Input: part model. Units: mm. Frame: model coordinates. Coordinates: 2 decimals unless noted, no trailing zeros. Loops run counter-clockwise (first coordinate to the right, second up) from the corner with the lowest first, then second, coordinate; pieces in that order, holes last. Notation, with made-up numbers: (34, 17.5) - (61, 17.5) arc R14 ccw to (61, 22.5) - close; hole circle Ø4 at (31.25, 3.25). An arc over 180 degrees is marked (long way). Use a Markdown table: item, result. Add a question column.
1. Ray query, L1, parallel to Y at x = 8.5, z = 2.05; L2, parallel to Y at x = -21.5, z = 2.85; L3, parallel to Y at x = 86, z = 1.1. Return the intervals inside material, ascending. Write a range as [from, to].
2. Section query B-B on x = 14. Return the cut outline in (y, z), then the cut area to 3 significant figures.
3. Section query D-D on x = -55.5. Return the cut outline in (y, z).
4. Contact query for flat-ended pins moving along their axis: P1, Ø1.5, axis at y = 71.5, z = 1, coming from the -X side; P2, Ø0.8, axis at x = 1, z = 1.5, coming from the +Y side. Output: stop coordinate, or through.
5. Section query C-C on x = -29. Return the cut outline in (y, z).
6. Draft query along Y for faces 1 (the face through (127.673, -116.235, 1.454)), 2 (the face through (76.285, 57.453, 1.454)), 3 (the face through (12, -34, 2.95)). Return one class per face: released by +Y, released by -Y, zero draft, split by the parting line, or undercut.
7. Section query A-A on z = 1.7. Return the cut outline in (x, y), then the cut area to 3 significant figures.
```python
from build123d import *

# Parameters (mm, degrees)
SKETCH1_W           = 15.45
SKETCH1_H           = 6.08
BOSS_EXTRUDE1_DEPTH = 2.95


with BuildPart() as part:
    # Sketch1 → Boss-Extrude1 (new body)
    with BuildSketch(Plane.XY):
        with BuildLine():
            Line((0.171167624, 69.469671818), (2.671167624, 69.469671818))
            Line((2.671167624, 69.469671818), (2.671167624, 75.099671818))
            Line((2.671167624, 75.099671818), (17.671167624, 75.099671818))
            Line((17.671167624, 75.099671818), (17.671167624, 69.469671818))
            Line((17.671167624, 69.469671818), (20.171167624, 69.469671818))
            ThreePointArc((20.171167624, 69.469671818), (77.092371221, 57.340494982), (135.171167624, 53.599671818))
            Line((135.171167624, 53.599671818), (135.171167624, -108.900328182))
            ThreePointArc((135.171167624, -108.900328182), (127.671167624, -116.400328182), (135.171167624, -123.900328182))
            Line((135.171167624, -123.900328182), (135.171167624, -146.400328182))
            Line((135.171167624, -146.400328182), (-114.828832376, -146.400328182))
            Line((-114.828832376, -146.400328182), (-114.828832376, 53.599671818))
            ThreePointArc((-114.828832376, 53.599671818), (-56.750035973, 57.340494982), (0.171167624, 69.469671818))
        make_face()
        with Locations((10.171167624, 50.559671818)):
            Rectangle(SKETCH1_W, SKETCH1_H, mode=Mode.SUBTRACT)
    extrude(amount=BOSS_EXTRUDE1_DEPTH)


solid = part.part
```
Resolved:
| question | item | result |
|---|---|---|
| 1 | L1 | [-146.4, 47.52], [53.6, 75.1] |
| 1 | L2 | [-146.4, 63.83] |
| 1 | L3 | [-146.4, 56.21] |
| 2 | outline | (-146.4, 0) - (47.52, 0) - (47.52, 2.95) - (-146.4, 2.95) - close; (53.6, 0) - (75.1, 0) - (75.1, 2.95) - (53.6, 2.95) - close |
| 2 | area | 635 mm² |
| 3 | outline | (-146.4, 0) - (57.52, 0) - (57.52, 2.95) - (-146.4, 2.95) - close |
| 4 | P1 | x = 2.67 |
| 4 | P2 | y = 69.47 |
| 5 | outline | (-146.4, 0) - (62.17, 0) - (62.17, 2.95) - (-146.4, 2.95) - close |
| 6 | face 1 | undercut |
| 6 | face 2 | released by +Y |
| 6 | face 3 | zero draft |
| 7 | outline | (-114.83, -146.4) - (135.17, -146.4) - (135.17, -123.9) arc R7.5 cw to (135.17, -108.9) - (135.17, 53.6) arc R400 cw to (20.17, 69.47) - (17.67, 69.47) - (17.67, 75.1) - (2.67, 75.1) - (2.67, 69.47) - (0.17, 69.47) arc R400 cw to (-114.83, 53.6) - close; hole (2.45, 47.52) - (17.9, 47.52) - (17.9, 53.6) - (2.45, 53.6) - close |
| 7 | area | 51,400 mm² |
